```python
from build123d import *

# Parameters (mm, degrees)
F0_W     = 304.8
F0_H     = 304.8
F1_DEPTH = 12.7
F2_R     = 9.525
F3_DEPTH = 12.7
F4_W     = 9.525
F4_H     = 38.1
F6_R     = 8.89
F7_DEPTH = 38.101


with BuildPart() as f1:
    # F0 (on Top) → F1 (new body)
    with BuildSketch(Plane.XY):
        Rectangle(F0_W, F0_H)
    extrude(amount=F1_DEPTH)

    # F2 (on Top) → F3 (cut, symmetric)
    with BuildSketch(Plane.XY):
        Circle(F2_R)
    extrude(amount=F3_DEPTH, both=True, mode=Mode.SUBTRACT)

    # F4 (on Front) → F5 (revolve)
    with BuildSketch(Plane.XZ):
        with Locations((4.7625, 19.05)):
            Rectangle(F4_W, F4_H)
    revolve(axis=Axis((0, 0, 19.05), (0, 0, 1)))

    # F6 (on Top) → F7 (cut, through all)
    with BuildSketch(Plane.XY):
        Circle(F6_R)
    extrude(amount=F7_DEPTH, mode=Mode.SUBTRACT)


solid = f1.part
```
CAD build for the part. Positions are in the model's coordinates, mm. A direction names the side the tool comes from. Coordinates: 2 decimals unless noted, no trailing zeros. Order: outer loops, then holes, each group sorted by start corner. A loop starts at its lowest first (then second) coordinate and runs counter-clockwise, first axis right, second up. Notation, with made-up numbers: M -5,-29 L 6,-29 A15 ccw 6,-19 Z; hole C 31.25,57.5 d7. An arc over 180 degrees is marked long. Write each question's results on one line, items separated by ' | '. Start each with the question number.
Q1. Which spindle directions (+Z, -Z, +X, -X, +Y, -Y) get a long thin tool onto all of the face, cutting with end or side? Do faces 1 (the flat face through (-152.4, -2, 6)), 2 (the cylindrical face through (-7.559, -5.796, 25.578)). Say none if no direction does.
Q2. Cut at A-A (x = 0). List the corners of the cut face in (y, z) (3 decimals), then the cut area to 3 significant figures.
Q3. Drill centre lines: probe 1 along Y at (x, z) = (0, 27) (3 decimals); probe 2 along Y at (x, z) = (0, 12); probe 3 along Z at (x, y) = (12.5, -16). Where is each one in solid material? Low to high. Write a range as from..to.
Q4. Flat gauge pin, fed straight in: P1, Ø6, axis at x = -5.5, z = 20.5, coming from the -Y side. Where does the tip first touch, or does it go through?
Q5. Cut at D-D (x = 105.5). List the corners of the cut face in (y, z).
Q6. Cut at C-C (z = 23). List the corners of the cut face in (x, y) (3 decimals).
Found:
1) face 1: +Z, -Z, -X, +Y, -Y | face 2: +Z
2) outline: M -152.4,0 L -8.89,0 L -8.89,38.1 L -9.525,38.1 L -9.525,12.7 L -152.4,12.7 Z; M 8.89,0 L 152.4,0 L 152.4,12.7 L 9.525,12.7 L 9.525,38.1 L 8.89,38.1 Z | area: 3,680 mm²
3) probe 1: -9.525..-8.89, 8.89..9.525 | probe 2: -152.4..-8.89, 8.89..152.4 | probe 3: 0..12.7
4) P1: y = -9.19
5) outline: M -152.4,0 L 152.4,0 L 152.4,12.7 L -152.4,12.7 Z
6) outline: C 0,0 d19.05; hole C 0,0 d17.78
